```python
from build123d import *

# Parameters (mm, degrees)
ESBO_O1_R                = 4
ESBO_O1_R_2              = 1.75
ESBO_O1_W                = 8
ESBO_O1_H                = 3
RESSALTO_EXTRUS_O1_DEPTH = 15
ESBO_O2_R                = 2.5
CORTE_EXTRUS_O1_DEPTH    = 15


with BuildPart() as part:
    # Esboço1 → Ressalto-extrusão1 (new body)
    with BuildSketch(Plane.XY):
        with BuildLine():
            Line((50, 0), (50, -10))
            ThreePointArc((50, -10), (42.588190451, -19.659258263), (31.339745962, -15))
            Line((31.339745962, -15), (-31.339745962, -15))
            ThreePointArc((-31.339745962, -15), (-42.588190451, -19.659258263), (-50, -10))
            Line((-50, -10), (-50, 0))
            Line((-50, 0), (50, 0))
        make_face()
        with Locations((-40, -10)):
            Circle(ESBO_O1_R, mode=Mode.SUBTRACT)
        with Locations(Location((40, -10, 0), (0, 0, 180))):
            Circle(ESBO_O1_R, mode=Mode.SUBTRACT)
        with Locations((10, -10)):
            Circle(ESBO_O1_R_2, mode=Mode.SUBTRACT)
        with Locations((-10, -10)):
            Circle(ESBO_O1_R_2, mode=Mode.SUBTRACT)
        with Locations((0, -3)):
            Rectangle(ESBO_O1_W, ESBO_O1_H, mode=Mode.SUBTRACT)
    extrude(amount=RESSALTO_EXTRUS_O1_DEPTH)

    # Esboço2 → Corte-extrusão1 (cut)
    with BuildSketch(Plane.XZ.offset(15)):
        with Locations((22.5, 7.5)):
            Circle(ESBO_O2_R)
        with Locations((-22.5, 7.5)):
            Circle(ESBO_O2_R)
    extrude(amount=-CORTE_EXTRUS_O1_DEPTH, mode=Mode.SUBTRACT)


solid = part.part
```
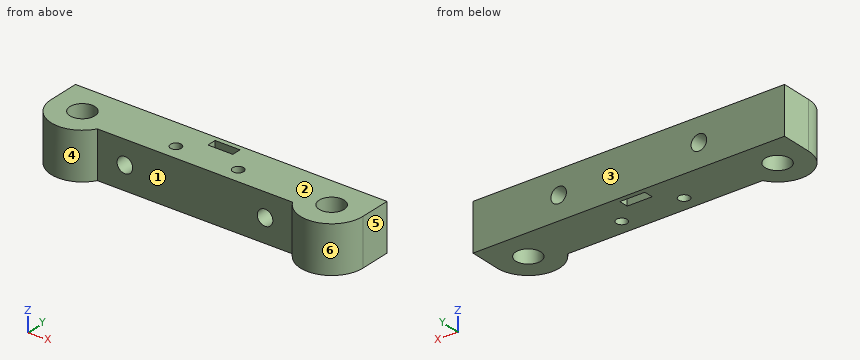
Geometry: final body of the model. Coordinates: model frame, mm. Face numbers are marked on the shaded views. A direction names the side the tool comes from. Round coordinates to 2 decimals unless told otherwise and drop trailing zeros. Write each loop counter-clockwise with the first axis right and the second up, starting at its lowest first coordinate (ties: lowest second). Pieces come first, ordered by that corner, then holes.
Item 1: Section query D-D (x = -10). Return loops of the section in (y, z), plus the area to 4 significant figures.
Item 2: Section query C-C (x = 21). Return loops of the section in (y, z).
Item 3: Mould query, pull axis X, two halves, no side actions, for the marked faces 3, 4, 5 and 6. Classes: +X half, -X half, draft (parallel to the pull), parting line (faces both ways), or undercut.
Item 4: Section query B-B (y = -2.75). Return loops of the section in (x, z).
Item 5: Set-up query: the marked faces 1 and 2. Return all of +Z, -Z, +X, -X, +Y, -Y with unobstructed straight access to the full face (end or side cutting, diameter ignored); none if empty.
Item 6: Pin query (flat end, axial travel): P1, Ø6, axis at x = 22.5, z = 7.5, coming from the -Y side; P2, Ø4, axis at x = 0, z = 8.5, coming from the +Y side. Return the tip coordinate at first contact, or that it passes through.
Item 7: Section query A-A (z = 6). Return loops of the section in (x, y), plus the area to 3 significant figures.
Item 8: Material intervals for L1, parallel to X at y = -3.5, z = 1; L2, parallel to Y at x = -40, z = 6.5; L3, parallel to Z at x = 22.5, y = -7, sorted ascending.
Completed:
1. outline: (-15, 0) - (-11.75, 0) - (-11.75, 15) - (-15, 15) - close; (-8.25, 0) - (0, 0) - (0, 15) - (-8.25, 15) - close
1. area: 172.5 mm2
2. outline: (-15, 0) - (0, 0) - (0, 5.5) - (-15, 5.5) - close; (-15, 9.5) - (0, 9.5) - (0, 15) - (-15, 15) - close
3. face 3: draft
3. face 4: undercut
3. face 5: +X half
3. face 6: undercut
4. outline: (-50, 0) - (-4, 0) - (-4, 15) - (-50, 15) - close; (4, 0) - (50, 0) - (50, 15) - (4, 15) - close; hole circle Ø5 at (-22.5, 7.5); hole circle Ø5 at (22.5, 7.5)
5. face 1: +Z, -Z, -Y
5. face 2: +Z, +X, -X, +Y, -Y
6. P1: stops at y = -15
6. P2: stops at y = 0
7. outline: (-50, -10) arc R10 ccw to (-31.34, -15) - (-24.5, -15) - (-24.5, 0) - (-50, 0) - close; (-20.5, -15) - (20.5, -15) - (20.5, 0) - (-20.5, 0) - close; (24.5, -15) - (31.34, -15) arc R10 ccw to (50, -10) - (50, 0) - (24.5, 0) - close; hole circle Ø8 at (-40, -10); hole circle Ø3.5 at (-10, -10); hole (-4, -4.5) - (4, -4.5) - (4, -1.5) - (-4, -1.5) - close; hole circle Ø3.5 at (10, -10); hole circle Ø8 at (40, -10)
7. area: 1,350 mm2
8. L1: x = -50 to -4, 4 to 50
8. L2: y = -20 to -14, -6 to 0
8. L3: z = 0 to 5, 10 to 15
